Check sheet for the modelled part. Datum: model origin and axes. Units: mm. A direction names the side the tool comes from. Round coordinates to 2 decimals unless told otherwise and drop trailing zeros. Loops run counter-clockwise (first coordinate to the right, second up) from the corner with the lowest first, then second, coordinate; pieces in that order, holes last. Notation, with made-up numbers: (-2.5, 66.25) - (41.5, 66.25) arc R14 cw to (41.5, 85.25) - close; hole circle Ø8 at (25.25, -9). An arc over 180 degrees is marked (long way). Put each result on its own line as item: value.
```python
from build123d import *

# Parameters (mm, degrees)
F1_DEPTH = 63.5
F0_W     = 25.4
F0_H     = 19.05
F0_H_2   = 4.7498
F0_H_3   = 4.7752
F2_DEPTH = 25.4


with BuildPart() as f1:
    # F0 (on Front) → F1 (new body, symmetric)
    with BuildSketch(Plane.XZ):
        Polygon((22.225, 9.525), (-41.275, 9.525), (-41.275, -9.525), (41.275, -9.525), (41.275, 9.525), align=None)
    extrude(amount=F1_DEPTH, both=True)

    # F0 (on Front) → F2 (join)
    with BuildSketch(Plane.XZ):
        with BuildLine():
            add(Edge.make_bspline(
                [(53.1596094472, 61.6964881046), (16.1985409417, 58.8323622572), (-40.681488346, 34.7288044556), (-41.275, 9.525)],
                knots=[3.9524583094, 3.9524583094, 3.9524583094, 3.9524583094, 111.5045361635, 111.5045361635, 111.5045361635, 111.5045361635], degree=3))
            Line((-41.275, 9.525), (22.225, 9.525))
            Line((22.225, 9.525), (22.225, 27.0002))
            ThreePointArc((22.225, 27.0002), (31.0816282149, 50.242308714), (53.1596094472, 61.6964881046))
        make_face()
        Polygon((22.225, 9.525), (-41.275, 9.525), (-41.275, -9.525), (41.275, -9.525), (41.275, 9.525), align=None)
        with BuildLine():
            Line((22.225, 27.0002), (22.225, 9.525))
            Line((22.225, 9.525), (41.275, 9.525))
            Line((41.275, 9.525), (41.275, 27.0002))
            ThreePointArc((41.275, 27.0002), (45.9246798487, 38.2255201513), (57.15, 42.8752))
            Line((57.15, 42.8752), (60.325, 42.8752))
            Line((60.325, 42.8752), (60.325, 61.9252))
            Line((60.325, 61.9252), (57.15, 61.9252))
            add(Edge.make_bspline(
                [(57.15, 61.9252), (55.849291913, 61.878313053), (54.5179010326, 61.8017425844), (53.1596094472, 61.6964881046)],
                knots=[0, 0, 0, 0, 3.9524583094, 3.9524583094, 3.9524583094, 3.9524583094], degree=3))
            ThreePointArc((53.1596094472, 61.6964881046), (31.0816282149, 50.242308714), (22.225, 27.0002))
        make_face()
        with BuildLine():
            ThreePointArc((57.15, 61.9252), (55.151530217, 61.8679751445), (53.1596094472, 61.6964881046))
            add(Edge.make_bspline(
                [(57.15, 61.9252), (55.849291913, 61.878313053), (54.5179010326, 61.8017425844), (53.1596094472, 61.6964881046)],
                knots=[0, 0, 0, 0, 3.9524583094, 3.9524583094, 3.9524583094, 3.9524583094], degree=3))
        make_face()
        with Locations((73.025, 52.4002)):
            Rectangle(F0_W, F0_H)
        with Locations((73.025, 64.3001)):
            Rectangle(F0_W, F0_H_2)
        with Locations((73.025, 40.4876)):
            Rectangle(F0_W, F0_H_3)
        Polygon((85.725, 66.675), (85.725, 61.9252), (85.725, 42.8752), (85.725, 38.1), (111.125, 38.1), (111.125, 66.675), align=None)
    extrude(amount=F2_DEPTH)


solid = f1.part
```
Item 1: Release check for a two-part mould opening along X. For faces 4 (the flat face through (-1, 1, -9.525)), 5 (the flat face through (60.325, -13, 64)), 6 (the flat face through (60.325, -13, 40)), 7 (the flat face through (41.275, 1, 0)) record: +X half, -X half, draft (parallel to the pull), parting line (faces both ways), or undercut.
Filled sheet:
face 4: draft
face 5: -X half
face 6: undercut
face 7: +X half
Item 2: Section check B-B on y = -41.5. Enter the section's corners in (x, z) (3 decimals).
Filled sheet:
outline: (-41.275, -9.525) - (41.275, -9.525) - (41.275, 9.525) - (-41.275, 9.525) - close
Item 3: Tool access check on faces 1 (the cylindrical face through (45.8, -12.5, 38.1)), 2 (the flat face through (85, -13, 38.1)), 3 (the flat face through (1, -45, 9.525)). Record the directions out of +Z, -Z, +X, -X, +Y, -Y that give a thin tool (end or side, any length) a straight path to the whole face; none if there is none.
Filled sheet:
face 1: -Z, +Y, -Y
face 2: -Z, +X, +Y, -Y
face 3: +Z, +X, -X, -Y
Item 4: Section check A-A on x = 100. Enter the section's corners in (y, z) (3 decimals).
Filled sheet:
outline: (-25.4, 38.1) - (0, 38.1) - (0, 66.675) - (-25.4, 66.675) - close
Item 5: Thickness scan on line 1 (Z direction, x = -0.5, y = 31) (3 decimals); line 2 (Y direction, x = -13, z = 41); line 3 (X direction, y = 13.5, z = 4) (3 decimals). Record the ranges inside material, lowest first. Write a range as from..to.
Filled sheet:
line 1: -9.525..9.525
line 2: -25.4..0
line 3: -41.275..41.275
Item 6: Go/stop test with flat-tipped pins: pin 1 (1.4 mm diameter, centred on y = -11.5, z = 41.5, fed in from -X); pin 2 (8 mm diameter, centred on x = 20, z = 44, fed in from -Y); pin 3 (3.5 mm diameter, centred on x = 59.5, y = -16.5, fed in from -Z). Record where each tip stops, or that it passes through.
Filled sheet:
pin 1: x = -13.66
pin 2: y = -25.4
pin 3: z = 38.1
